Could you check a few things on this model? Use its own coordinates, in mm. Face numbers are marked on the shaded views. A direction names the side the tool comes from. Give positions to 0.01 mm unless a question says otherwise; leave off trailing zeros. Order: outer loops, then holes, each group sorted by start corner. A loop starts at its lowest first (then second) coordinate and runs counter-clockwise, first axis right, second up. Notation, with made-up numbers: (11.25, 10.5) -> (39.25, 10.5) arc R28 ccw to (39.25, 41.5) -> close; hole circle Ø8 at (44, 21.5). An arc over 180 degrees is marked (long way). One line per item, written item: value.
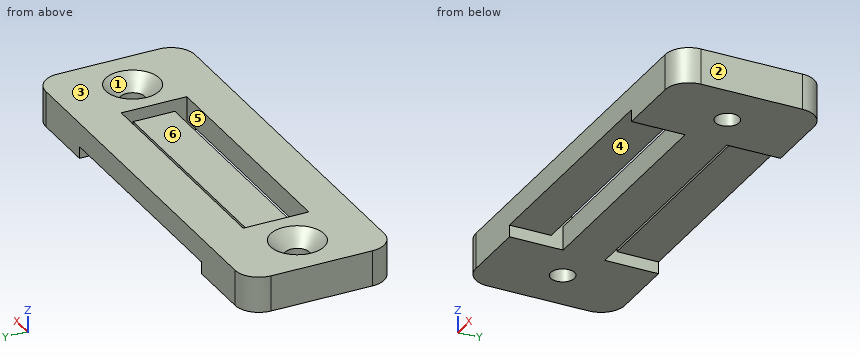
```python
from build123d import *

# Parameters (mm, degrees)
CYLINDER001_R     = 2
CYLINDER001_DEPTH = 10
CYLINDER003_R     = 2
CYLINDER003_DEPTH = 10
BOX006_W          = 40
BOX006_H          = 11
BOX006_DEPTH      = 10
BOX001_W          = 40
BOX001_H          = 25
BOX001_DEPTH      = 2
BOX_W             = 70
BOX_H             = 25
BOX_DEPTH         = 6
CHAMFER_SIZE      = 2.49
FILLET_R          = 4
BOX003_W          = 40
BOX003_H          = 7
BOX003_DEPTH      = 4


with BuildPart() as screwhole002:
    # Cylinder001 → Cylinder001 (new body)
    with BuildSketch(Plane(origin=(-27, -7.5, 0), x_dir=(1, 0, 0), z_dir=(0, 0, 1))):
        Circle(CYLINDER001_R)
    extrude(amount=CYLINDER001_DEPTH)


with BuildPart() as screwholes:
    # Cylinder003 → Cylinder003 (new body)
    with BuildSketch(Plane(origin=(27, -7.5, 0), x_dir=(1, 0, 0), z_dir=(0, 0, 1))):
        Circle(CYLINDER003_R)
    extrude(amount=CYLINDER003_DEPTH)

    # Fusion001: union ScrewHole002
    add(screwhole002.part)


with BuildPart() as cube001:
    # Box006 → Box006 (new body)
    with BuildSketch(Plane(origin=(-20, -13, 0), x_dir=(1, 0, 0), z_dir=(0, 0, 1))):
        with Locations((20, 5.5)):
            Rectangle(BOX006_W, BOX006_H)
    extrude(amount=BOX006_DEPTH)


with BuildPart() as cube:
    # Box001 → Box001 (new body)
    with BuildSketch(Plane(origin=(-20, -20, 0), x_dir=(1, 0, 0), z_dir=(0, 0, 1))):
        with Locations((20, 12.5)):
            Rectangle(BOX001_W, BOX001_H)
    extrude(amount=BOX001_DEPTH)


with BuildPart() as fillet_body:
    # Box → Box (new body)
    with BuildSketch(Plane(origin=(-35, -20, 0), x_dir=(1, 0, 0), z_dir=(0, 0, 1))):
        with Locations((35, 12.5)):
            Rectangle(BOX_W, BOX_H)
    extrude(amount=BOX_DEPTH)

    # Cut: cut Cube
    add(cube.part, mode=Mode.SUBTRACT)

    # Cut001: cut Cube001
    add(cube001.part, mode=Mode.SUBTRACT)

    # Cut002: cut ScrewHoles
    add(screwholes.part, mode=Mode.SUBTRACT)

    # Chamfer
    chamfer_edges = [fillet_body.edges().sort_by_distance(p)[0] for p in [
        (-29, -7.5, 6),
        (25, -7.5, 6),
    ]]
    chamfer(chamfer_edges, length=CHAMFER_SIZE)

    # Fillet
    fillet_edges = [fillet_body.edges().sort_by_distance(p)[0] for p in [
        (-35, -20, 3),
        (-35, 5, 3),
        (35, 5, 3),
        (35, -20, 3),
    ]]
    fillet(fillet_edges, radius=FILLET_R)


with BuildPart() as fusion:
    # Box003 → Box003 (new body)
    with BuildSketch(Plane(origin=(-20, -11, 0), x_dir=(1, 0, 0), z_dir=(0, 0, 1))):
        with Locations((20, 3.5)):
            Rectangle(BOX003_W, BOX003_H)
    extrude(amount=BOX003_DEPTH)

    # Fusion: union Fillet body
    add(fillet_body.part)


solid = fusion.part
```
1) Suppose I cut it at B-B, the plane y = -7.5. Write out the boundary of the cut face in (x, z), then the cut area to 3 significant figures.
Answer below:
outline: (-35, 0) -> (-29, 0) -> (-29, 3.51) -> (-31.49, 6) -> (-35, 6) -> close; (-25, 0) -> (25, 0) -> (25, 3.51) -> (22.51, 6) -> (20, 6) -> (20, 4) -> (-20, 4) -> (-20, 6) -> (-22.51, 6) -> (-25, 3.51) -> close; (29, 0) -> (35, 0) -> (35, 6) -> (31.49, 6) -> (29, 3.51) -> close
area: 280 mm2
2) Suppose I cut it at D-D, the plane z = 5.2. Write out the boundary of the cut face in (x, y).
Answer below:
outline: (-35, -16) arc R4 ccw to (-31, -20) -> (31, -20) arc R4 ccw to (35, -16) -> (35, 1) arc R4 ccw to (31, 5) -> (-31, 5) arc R4 ccw to (-35, 1) -> close; hole circle Ø7.38 at (-27, -7.5); hole (-20, -13) -> (20, -13) -> (20, -2) -> (-20, -2) -> close; hole circle Ø7.38 at (27, -7.5)
3) If I drill on line 1 along Y through (x, z) = (16.5, 3.6); line 2 along X through (y, z) = (-7.5, 2.1); line 3 along Y through (x, z) = (27, 1.2), over which ranges is the centre line in solid material (lowest first)?
Answer below:
line 1: y = -20 to -13, -11 to -4, -2 to 5
line 2: x = -35 to -29, -25 to 25, 29 to 35
line 3: y = -20 to -9.5, -5.5 to 5
4) For the marked faces 4, 5 and 6, which set-ups out of +Z, -Z, +X, -X, +Y, -Y let a thin tool reach every point of the face, with its end or its side?
Answer below:
face 4: -Z, -Y
face 5: +Z, -Z
face 6: +Z
5) For P1, Ø5.5, axis at x = -2, y = -15.5, coming from the -Z side; P2, Ø5.5, axis at x = 4.5, y = -9, coming from the +Z side; P3, Ø6.5, axis at x = -27, y = -7.5, coming from the +Z side, each with a flat end and sliding along its axis, tell me the tip position at first contact or that it passes through.
Answer below:
P1: stops at z = 2
P2: stops at z = 4
P3: stops at z = 4.76
6) Suppose I cut it at C-C, the plane x = 27. Write out the boundary of the cut face in (y, z).
Answer below:
outline: (-20, 0) -> (-9.5, 0) -> (-9.5, 3.51) -> (-11.99, 6) -> (-20, 6) -> close; (-5.5, 0) -> (5, 0) -> (5, 6) -> (-3.01, 6) -> (-5.5, 3.51) -> close
7) We'd pull the mould along X, two halves only. Please class the marked faces 1, 2 and 3: +X half, -X half, draft (parallel to the pull), parting line (faces both ways), or undercut.
Answer below:
face 1: undercut
face 2: +X half
face 3: draft
8) Suppose I cut it at A-A, the plane x = 3. Write out the boundary of the cut face in (y, z).
Answer below:
outline: (-20, 2) -> (-13, 2) -> (-13, 6) -> (-20, 6) -> close; (-11, 0) -> (-4, 0) -> (-4, 4) -> (-11, 4) -> close; (-2, 2) -> (5, 2) -> (5, 6) -> (-2, 6) -> close
